```python
from build123d import *

# Parameters (mm, degrees)
SKETCH1_W           = 65
SKETCH1_H           = 65
BOSS_EXTRUDE1_DEPTH = 3
SKETCH2_R           = 2.5
BOSS_EXTRUDE2_DEPTH = 17
CUT_EXTRUDE1_DEPTH  = 21
FILLET1_R           = 0.5


with BuildPart() as part:
    # Sketch1 → Boss-Extrude1 (new body)
    with BuildSketch(Plane(origin=(0, 0, 0), x_dir=(1, 0, 0), z_dir=(0, 1, 0))):
        Rectangle(SKETCH1_W, SKETCH1_H)
    extrude(amount=BOSS_EXTRUDE1_DEPTH)

    # Sketch2 → Boss-Extrude2 (add)
    with BuildSketch(Plane(origin=(0, 3, 0), x_dir=(1, 0, 0), z_dir=(0, 1, 0))):
        with Locations((-19.5, 19.5)):
            Circle(SKETCH2_R)
        with Locations((19.5, 19.5)):
            Circle(SKETCH2_R)
        with Locations((-19.5, -19.5)):
            Circle(SKETCH2_R)
        with Locations((19.5, -19.5)):
            Circle(SKETCH2_R)
    extrude(amount=BOSS_EXTRUDE2_DEPTH)

    # Sketch3 → Cut-Extrude1 (cut, through all)
    with BuildSketch(Plane.XZ):
        with BuildLine():
            Line((-19.335806009, 4.005402362), (20.966240956, 4.005402362))
            ThreePointArc((20.966240956, 4.005402362), (24.971643318, 0), (20.966240956, -4.005402362))
            Line((20.966240956, -4.005402362), (-19.335806009, -4.005402362))
            ThreePointArc((-19.335806009, -4.005402362), (-23.34120837, 0), (-19.335806009, 4.005402362))
        make_face()
    extrude(amount=-CUT_EXTRUDE1_DEPTH, mode=Mode.SUBTRACT)

    # Fillet1
    fillet1_edges = [part.edges().sort_by_distance(p)[0] for p in [
        (-32.5, 3, 0),
        (-22, 20, -19.5),
        (0, 3, 32.5),
        (17, 20, -19.5),
        (-22, 20, 19.5),
        (17, 20, 19.5),
        (32.5, 3, 0),
        (0, 0, 32.5),
        (-32.5, 0, 0),
        (0, 0, -32.5),
        (32.5, 0, 0),
        (0, 3, -32.5),
    ]]
    fillet(fillet1_edges, radius=FILLET1_R)


solid = part.part
```
Can you work these out from the model? Positions are in its coordinate system, mm. A direction names the side the tool comes from. Coordinates: 2 decimals unless noted, no trailing zeros. Loops run counter-clockwise (first coordinate to the right, second up) from the corner with the lowest first, then second, coordinate; pieces in that order, holes last. Notation, with made-up numbers: (41.5, -5.75) -> (93.5, -5.75) arc R19 ccw to (93.5, 20.25) -> close; hole circle Ø11 at (47, 59.5). An arc over 180 degrees is marked (long way). Put each result on its own line as item: value. Start each with the question number.
Q1. I'm going to push a flat-ended pin straight in: P1, Ø1.5, axis at x = 18, y = 18, coming from the +Z side. Where does the tip first touch, or does it pass through?
Q2. I want a section at D-D (z = -19.5). Write out the boundary of the cut face in (x, y), plus the area to 3 significant figures.
Q3. For faces 4 (the face through (19, 20, -20)), 5 (the face through (17.66, 11.13, -21.19)), 6 (the face through (-23.34, 1.48, -0.09)), which set-ups out of +Z, -Z, +X, -X, +Y, -Y let a thin tool reach every point of the face, with its end or its side?
Q4. Thinking about a two-plate mould opening in Z: for faces 1 (the face through (0, 1, 32.5)), 2 (the face through (0, 0, -8)), 3 (the face through (1, 1, -4.005)), which applies, pulls with the +Z half, pulls with the -Z half, needs draft (parallel to the pull), parting line crosses it, or undercut?
Q5. I want a section at A-A (x = -7). Write out the boundary of the cut face in (y, z).
Q6. If I drill on line 1 (Z direction, x = 19, y = 2.25); line 2 (X direction, y = 14.75, z = -18); line 3 (Y direction, x = 24, z = 9), over which ranges is the centre line in solid material (lowest first)? Write a range as [from, to].
Q7. I want a section at B-B (z = 0). Write out the boundary of the cut face in (x, y).
Q8. I want a section at C-C (x = 19.5). Write out the boundary of the cut face in (y, z), plus the area to 3 significant figures.
Taken from the geometry:
1. P1: stops at z = 21.88
2. outline: (-32.5, 0.5) arc R0.5 ccw to (-32, 0) -> (32, 0) arc R0.5 ccw to (32.5, 0.5) -> (32.5, 2.5) arc R0.5 ccw to (32, 3) -> (22, 3) -> (22, 19.5) arc R0.5 ccw to (21.5, 20) -> (17.5, 20) arc R0.5 ccw to (17, 19.5) -> (17, 3) -> (-17, 3) -> (-17, 19.5) arc R0.5 ccw to (-17.5, 20) -> (-21.5, 20) arc R0.5 ccw to (-22, 19.5) -> (-22, 3) -> (-32, 3) arc R0.5 ccw to (-32.5, 2.5) -> close
2. area: 365 mm2
3. face 4: +Z, -Z, +X, -X, +Y
3. face 5: +Y
3. face 6: +Y, -Y
4. face 1: pulls with the +Z half
4. face 2: needs draft
4. face 3: undercut
5. outline: (0, -32) arc R0.5 ccw to (0.5, -32.5) -> (2.5, -32.5) arc R0.5 ccw to (3, -32) -> (3, -4.01) -> (0, -4.01) -> close; (0, 4.01) -> (3, 4.01) -> (3, 32) arc R0.5 ccw to (2.5, 32.5) -> (0.5, 32.5) arc R0.5 ccw to (0, 32) -> close
6. line 1: z = [-32.5, -4.01], [4.01, 32.5]
6. line 2: x = [-21.5, -17.5], [17.5, 21.5]
6. line 3: y = [0, 3]
7. outline: (-32.5, 0.5) arc R0.5 ccw to (-32, 0) -> (-23.34, 0) -> (-23.34, 3) -> (-32, 3) arc R0.5 ccw to (-32.5, 2.5) -> close; (24.97, 0) -> (32, 0) arc R0.5 ccw to (32.5, 0.5) -> (32.5, 2.5) arc R0.5 ccw to (32, 3) -> (24.97, 3) -> close
8. outline: (0, -32) arc R0.5 ccw to (0.5, -32.5) -> (2.5, -32.5) arc R0.5 ccw to (3, -32) -> (3, -22) -> (19.5, -22) arc R0.5 ccw to (20, -21.5) -> (20, -17.5) arc R0.5 ccw to (19.5, -17) -> (3, -17) -> (3, -4.01) -> (0, -4.01) -> close; (0, 4.01) -> (3, 4.01) -> (3, 17) -> (19.5, 17) arc R0.5 ccw to (20, 17.5) -> (20, 21.5) arc R0.5 ccw to (19.5, 22) -> (3, 22) -> (3, 32) arc R0.5 ccw to (2.5, 32.5) -> (0.5, 32.5) arc R0.5 ccw to (0, 32) -> close
8. area: 341 mm2
